Here's how the part is built. I have some questions about the finished solid (model axes, mm). A direction names the side the tool comes from. Round coordinates to 2 decimals unless told otherwise and drop trailing zeros. Write each loop counter-clockwise with the first axis right and the second up, starting at its lowest first coordinate (ties: lowest second). Pieces come first, ordered by that corner, then holes. Notation, with made-up numbers: M -37.5,-18 L -32.5,-18 A20 cw -32.5,16 Z; hole C -38.75,0.25 d1. An arc over 180 degrees is marked long. Write item = value, one per line. Start each with the question number.
(1) I need wall thicknesses on line 1 along Z through (x, y) = (4, 5.75); line 2 along Z through (x, y) = (4.25, 0.5); line 3 along Y through (x, z) = (0.25, -119). Which ranges of each line are inside material? Lowest first, please.
(2) Will these pins go through, and if not, where does the flat tip stop? pin 1 Ø8 at (x, z) = (5.5, -34.5) entering from -Y; pin 2 Ø2 at (x, z) = (4, -117.5) entering from +Y; pin 3 Ø6 at (x, y) = (-6, -1.5) entering from -Z; pin 4 Ø5 at (x, z) = (6, -91) entering from +Y.
(3) I want a section at B-B (z = -117.5). List the corners of the cut face in (x, y) for me.
(4) On a 3-axis mill with a long thin cutter (end or side, diameter ignored), from which of +Z, -Z, +X, -X, +Y, -Y can I reach the whole of each face in a straight line? I mean faces 1 (the cylindrical face through (-1.08, -4.88, -53.24)), 2 (the flat face through (0, -8.001, 3)). Say none if no direction works.
Solid Edge part; units mm, degrees
sketch "Sketch1" plane through (0, 0, 0) normal (0, 0, 1) x (1, 0, 0)
  circle A0 centre (0, 0) radius 9.2812
extrude "Protrusion1" add sketch "Sketch1" along normal blind 6.604
sketch "Sketch2" plane through (0, 0, 0) normal (0, 0, -1) x (1, 0, 0)
  circle A0 centre (0, 0) radius 5
extrude "Protrusion2" add sketch "Sketch2" along normal blind 140
sketch "Sketch3" plane through (0, 0, -140) normal (0, 0, -1) x (1, 0, 0)
  circle A0 centre (0, 0) radius 4.9997
extrude "Cutout1" cut sketch "Sketch3" against normal blind 32.004 flip side to cut
chamfer "Chamfer_1" distance 0.75 angle 45 1 edges at (-4.9997, 0, -140)
sketch "Sketch4" plane through (0, 0, 6.604) normal (0, 0, 1) x (1, 0, 0)
  line L0 (-4.7036, 8.001) -> (4.7036, 8.001)
extrude "Cutout2" cut sketch "Sketch4" against normal up to next material side at (0, 8.051, 6.604)
pattern_circular "Pattern1" count 6 over 360 about axis through (0, 0, 6.604) along (0, 0, 1) of "Cutout2"
properties part number "118010" material "Stainless Steel, 304"
Returned:
q1.line_1 = 0 to 6.6
q1.line_2 = -139.97 to 6.6
q1.line_3 = -4.99 to 4.99
q2.pin_1 = -4.77
q2.pin_2 = 4
q2.pin_3 = -140
q2.pin_4 = 3.57
q3.outline = C 0,0 d10
q4.face_1 = -Z
q4.face_2 = +Z, -Z, +X, -X, -Y
